from build123d import *

# Parameters (mm, degrees)
SKETCH1_W           = 31.75
SKETCH1_H           = 101.6
SKETCH1_R           = 3.175
BOSS_EXTRUDE1_DEPTH = 6.35
SKETCH2_R           = 2.38125
CUT_EXTRUDE1_DEPTH  = 107.634633211
FILLET1_R           = 6.35


with BuildPart() as part:
    # Sketch1 → Boss-Extrude1 (new body)
    with BuildSketch(Plane.XY):
        with Locations((15.875, 50.8)):
            Rectangle(SKETCH1_W, SKETCH1_H)
        with Locations((25.4, 88.9)):
            Circle(SKETCH1_R, mode=Mode.SUBTRACT)
        with BuildLine():
            ThreePointArc((6.941258846, 98.129370577), (7.844693943, 78.050224174), (25.4, 68.2625))
            ThreePointArc((25.4, 68.2625), (26.9875, 69.85), (25.4, 71.4375))
            ThreePointArc((25.4, 71.4375), (10.545510259, 79.719420455), (9.781065177, 96.709467411))
            ThreePointArc((9.781065177, 96.709467411), (9.071113594, 98.83932216), (6.941258846, 98.129370577))
        make_face(mode=Mode.SUBTRACT)
    extrude(amount=BOSS_EXTRUDE1_DEPTH)

    # Sketch2 → Cut-Extrude1 (cut, through all)
    with BuildSketch(Plane.XY.offset(6.35)):
        with Locations((4.7625, 25.4)):
            Circle(SKETCH2_R)
        with Locations((26.9875, 25.4)):
            Circle(SKETCH2_R)
        with Locations((4.7625, 12.7)):
            Circle(SKETCH2_R)
        with Locations((26.9875, 12.7)):
            Circle(SKETCH2_R)
    extrude(amount=-CUT_EXTRUDE1_DEPTH, mode=Mode.SUBTRACT)

    # Fillet1
    fillet1_edges = [part.edges().sort_by_distance(p)[0] for p in [
        (0, 101.6, 3.175),
        (31.75, 101.6, 3.175),
    ]]
    fillet(fillet1_edges, radius=FILLET1_R)


solid = part.part
CAD build for the part. Positions are in the model's coordinates, mm. A direction names the side the tool comes from. Give positions to 0.01 mm unless a question says otherwise; leave off trailing zeros. Loops run counter-clockwise (first coordinate to the right, second up) from the corner with the lowest first, then second, coordinate; pieces in that order, holes last. Notation, with made-up numbers: M 71.25,65 L 109.25,65 A21 ccw 109.25,70 Z; hole C -29,53 d1. An arc over 180 degrees is marked long. One line per question, with ' | ' between items. Start each with the question number.
1. Saw through at C-C on z = 2.5. State how many separate pieces and enclosed holes the cut face has, plus the area to 3 significant figures.
2. Saw through at D-D on y = 69.85. Give the cut face in (x, z), plus the area to 3 significant figures.
3. Two-plate mould, pull along X, no slides. Class faces 1 (the face through (29.84, 99.79, 3.22)), 2 (the face through (1.81, 99.69, 3.22)), 3 (the face through (24.71, 85.8, 3.13)): pulls with the +X half, pulls with the -X half, needs draft (parallel to the pull), parting line crosses it, or undercut.
4. 3-axis set-ups, long thin cutter, end or side, ignore diameter. For faces 4 (the face through (16, 101.6, 3)), 5 (the face through (26.987, 69.815, 3.131)): which of +Z, -Z, +X, -X, +Y, -Y reach the whole face in a straight line?
5. Saw through at A-A on y = 25.4. Give the cut face in (x, z).
6. Probe L1, parallel to Y at x = 26, z = 4; L2, parallel to Y at x = 3.5, z = 1.5; L3, parallel to X at y = 89.5, z = 4.5. List the from-to ranges inside material, lowest first. Write a range as from..to.
7. Saw through at B-B on x = 19. Give the cut face in (y, z), plus the area to 3 significant figures.
Result sheet:
1) separate pieces: 1 | enclosed holes: 6 | area: 2,970 mm^2
2) outline: M 0,0 L 17.46,0 L 17.46,6.35 L 0,6.35 Z; M 26.99,0 L 31.75,0 L 31.75,6.35 L 26.99,6.35 Z | area: 141 mm^2
3) face 1: pulls with the +X half | face 2: pulls with the -X half | face 3: undercut
4) face 4: +Z, -Z, +X, -X, +Y | face 5: +Z, -Z
5) outline: M 0,0 L 2.38,0 L 2.38,6.35 L 0,6.35 Z; M 7.14,0 L 24.61,0 L 24.61,6.35 L 7.14,6.35 Z; M 29.37,0 L 31.75,0 L 31.75,6.35 L 29.37,6.35 Z
6) L1: y = 0..10.53, 14.87..23.23, 27.57..68.38, 71.32..85.78, 92.02..101.57 | L2: y = 0..10.68, 14.72..23.38, 27.42..100.92 | L3: x = 0..4.77, 7.95..22.28, 28.52..31.75
7) outline: M 0,0 L 69.28,0 L 69.28,6.35 L 0,6.35 Z; M 72.65,0 L 101.6,0 L 101.6,6.35 L 72.65,6.35 Z | area: 624 mm^2
